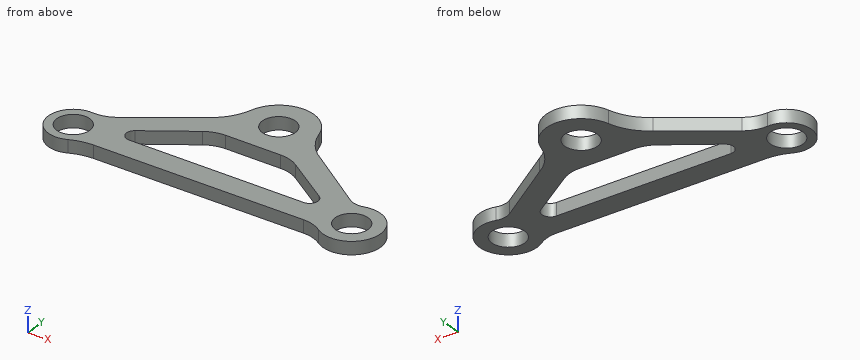
from build123d import *

# Parameters (mm, degrees)
SKETCH1_R           = 8
BOSS_EXTRUDE5_DEPTH = 6.2


with BuildPart() as part:
    # Sketch1 → Boss-Extrude5 (new body)
    with BuildSketch(Plane.XY):
        with BuildLine():
            Line((56.326485312, -30.684522316), (27.5, -10.5))
            ThreePointArc((27.5, -10.5), (20.534538743, -4.128471677), (16.428279646, 4.371684787))
            ThreePointArc((16.428279646, 4.371684787), (0, 17), (-16.428279646, 4.371684787))
            ThreePointArc((-16.428279646, 4.371684787), (-20.534538743, -4.128471677), (-27.5, -10.5))
            Line((-27.5, -10.5), (-56.326485312, -30.684522316))
            ThreePointArc((-56.326485312, -30.684522316), (-61.265597018, -33.006583144), (-66.697832686, -33.533466974))
            ThreePointArc((-66.697832686, -33.533466974), (-79.395490057, -47.670549132), (-62.498849309, -56.364864865))
            ThreePointArc((-62.498849309, -56.364864865), (-57.322133361, -54.598377325), (-51.885147908, -54))
            Line((-51.885147908, -54), (50.093284326, -54))
            ThreePointArc((50.093284326, -54), (54.937524893, -54.750956314), (59.327038829, -56.933333333))
            ThreePointArc((59.327038829, -56.933333333), (81.19137471, -47.945254568), (63.752518972, -31.985271674))
            ThreePointArc((63.752518972, -31.985271674), (59.894931525, -32.160256826), (56.326485312, -30.684522316))
        make_face()
        with Locations(Location((67.406574019, -45.5, 0), (0, 0, 180))):
            Circle(SKETCH1_R, mode=Mode.SUBTRACT)
        with Locations(Location((0, 0, 0), (0, 0, 180))):
            Circle(SKETCH1_R, mode=Mode.SUBTRACT)
        with Locations(Location((-67.593425981, -45.5, 0), (0, 0, 180))):
            Circle(SKETCH1_R, mode=Mode.SUBTRACT)
        with BuildLine():
            Line((13.373633763, -17.668465774), (-13.446021539, -17.613430543))
            ThreePointArc((-13.446021539, -17.613430543), (-18.208444632, -18.31519172), (-22.557597192, -20.378687414))
            Line((-22.557597192, -20.378687414), (-44.744358674, -35.277702309))
            ThreePointArc((-44.744358674, -35.277702309), (-46.370360965, -39.839621324), (-42.483173297, -42.728351249))
            Line((-42.483173297, -42.728351249), (42.307503535, -42.902337904))
            ThreePointArc((42.307503535, -42.902337904), (46.206513764, -40.029584072), (44.599245091, -35.46103039))
            Line((44.599245091, -35.46103039), (22.473807978, -20.471098353))
            ThreePointArc((22.473807978, -20.471098353), (18.133148836, -18.389767499), (13.373633763, -17.668465774))
        make_face(mode=Mode.SUBTRACT)
    extrude(amount=BOSS_EXTRUDE5_DEPTH)


solid = part.part
Geometry: final body of the model. Coordinates: model frame, mm. Coordinates: 2 decimals unless noted, no trailing zeros. Order: outer loops, then holes, each group sorted by start corner. A loop starts at its lowest first (then second) coordinate and runs counter-clockwise, first axis right, second up.
1) Section B-B (x = -5.5). Return loops of the section in (y, z), then the cut area to 3 significant figures.
Result sheet:
outline: (-54, 0) - (-42.8, 0) - (-42.8, 6.2) - (-54, 6.2) - close; (-17.63, 0) - (-5.81, 0) - (-5.81, 6.2) - (-17.63, 6.2) - close; (5.81, 0) - (16.09, 0) - (16.09, 6.2) - (5.81, 6.2) - close
area: 206 mm2
2) Ray query, probe 1 along X at (y, z) = (-45.5, 1.5); probe 2 along Y at (x, z) = (-5, 4.5) (3 decimals); probe 3 along Y at (x, z) = (-2, 5.5). Return the intervals inside material, ascending.
Result sheet:
probe 1: x = -79.59 to -75.59, -59.59 to 59.41, 75.41 to 81.41
probe 2: y = -54 to -42.805, -17.631 to -6.245, 6.245 to 16.248
probe 3: y = -54 to -42.81, -17.64 to -7.75, 7.75 to 16.88
3) Section C-C (y = -26). Return loops of the section in (x, z).
Result sheet:
outline: (-49.64, 0) - (-30.93, 0) - (-30.93, 6.2) - (-49.64, 6.2) - close; (30.63, 0) - (49.64, 0) - (49.64, 6.2) - (30.63, 6.2) - close
4) Section D-D (x = -32.5). Return loops of the section in (y, z), then the cut area to 3 significant figures.
Result sheet:
outline: (-54, 0) - (-42.75, 0) - (-42.75, 6.2) - (-54, 6.2) - close; (-27.06, 0) - (-14, 0) - (-14, 6.2) - (-27.06, 6.2) - close
area: 151 mm2
5) First-contact query: P1, Ø1, axis at x = 43, z = 3, coming from the -Y side; P2, Ø2, axis at y = -20, z = 2.5, coming from the -X side; P3, Ø1, axis at x = -32.5, z = 5.5, coming from the +Y side. Flat tips, straight axial feed; report the tip coordinate or a pass-through.
Result sheet:
P1: stops at y = -54
P2: stops at x = -42.5
P3: stops at y = -13.65
6) Section A-A (y = -45.5). Return loops of the section in (x, z).
Result sheet:
outline: (-79.59, 0) - (-75.59, 0) - (-75.59, 6.2) - (-79.59, 6.2) - close; (-59.59, 0) - (59.41, 0) - (59.41, 6.2) - (-59.59, 6.2) - close; (75.41, 0) - (81.41, 0) - (81.41, 6.2) - (75.41, 6.2) - close
